from build123d import *

# Parameters (mm, degrees)
PAD003_DEPTH = 5


with BuildPart() as part:
    # Sketch003 → Pad003 (new body)
    with BuildSketch(Plane.XY):
        with BuildLine():
            add(Edge.make_bspline(
                [(363.489628, -162.788216), (241.851853, -141.268772)],
                knots=[0, 0, 350.154309, 350.154309], degree=1))
            add(Edge.make_bspline(
                [(363.489628, -162.788216), (313.712684, -196.302104)],
                knots=[0, 0, 170.100588, 170.100588], degree=1))
            add(Edge.make_bspline(
                [(313.712684, -196.302104), (350.895461, -251.511825)],
                knots=[0, 0, 188.683359, 188.683359], degree=1))
            add(Edge.make_bspline(
                [(294.839074, -299.172102), (350.895461, -251.511825)],
                knots=[0, 0, 208.569461, 208.569461], degree=1))
            add(Edge.make_bspline(
                [(210.560464, -176.017382), (294.839074, -299.172102)],
                knots=[0, 0, 423.017754, 423.017754], degree=1))
            add(Edge.make_bspline(
                [(241.851853, -141.268772), (210.560464, -176.017382)],
                knots=[0, 0, 132.55165, 132.55165], degree=1))
        make_face()
        with BuildLine():
            add(Edge.make_bspline(
                [(323.661017, -216.445715), (312.442684, -223.995159)],
                knots=[0, 0, 38.330145, 38.330145], degree=1))
            add(Edge.make_bspline(
                [(312.442684, -223.995159), (312.724907, -224.383215)],
                knots=[0, 0, 1.360147, 1.360147], degree=1))
            add(Edge.make_bspline(
                [(312.724907, -224.383215), (323.907962, -216.869048)],
                knots=[0, 0, 38.19136, 38.19136], degree=1))
            add(Edge.make_bspline(
                [(323.907962, -216.869048), (323.661017, -216.445715)],
                knots=[0, 0, 1.389244, 1.389244], degree=1))
        make_face(mode=Mode.SUBTRACT)
    extrude(amount=PAD003_DEPTH)


solid = part.part
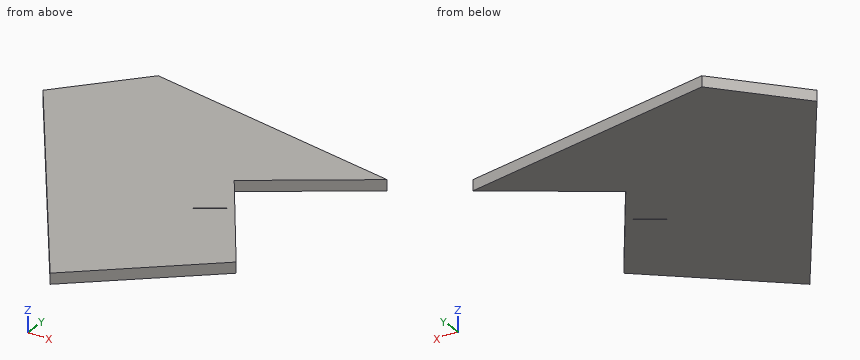
CAD build for the part. Positions are in the model's coordinates, mm. Give positions to 0.01 mm unless a question says otherwise; leave off trailing zeros. One line per question, with ' | ' between items. Start each with the question number.
1. Saw through at A-A on x = 321. State how many separate pieces and enclosed holes the cut face has, plus the area to 3 significant figures.
2. Flat gauge pins, fed straight in: pin 1 (1.5 mm diameter, centred on y = -170, z = 3, fed in from +X); pin 2 (1.5 mm diameter, centred on y = -255, z = 3.5, fed in from +X); pin 3 (1 mm diameter, centred on x = 288.5, z = 2.5, fed in from +Y). Where does each tip first touch, or does it go through?
3. Probe L1, parallel to Y at x = 316, z = 3.15; L2, parallel to Y at x = 329, z = 2; L3, parallel to Y at x = 343, z = 3.05. List the from-to ranges inside material, lowest first. Write a range as from..to.
Result sheet:
1) separate pieces: 3 | enclosed holes: 0 | area: 527 mm^2
2) pin 1: stops at x = 353.89 | pin 2: stops at x = 347.67 | pin 3: stops at y = -149.43
3) L1: y = -281.18..-222.18, -221.6..-199.7, -194.76..-154.39 | L2: y = -270.13..-219, -186.01..-156.69 | L3: y = -258.22..-239.79, -176.58..-159.16
